Geometry check sheet. Reference: drawing and pictorial views, mm from the part's lowest x, y, z. A direction names the side the tool comes from. Coordinates: 2 decimals unless noted, no trailing zeros. Loops run counter-clockwise (first coordinate to the right, second up) from the corner with the lowest first, then second, coordinate; pieces in that order, holes last.
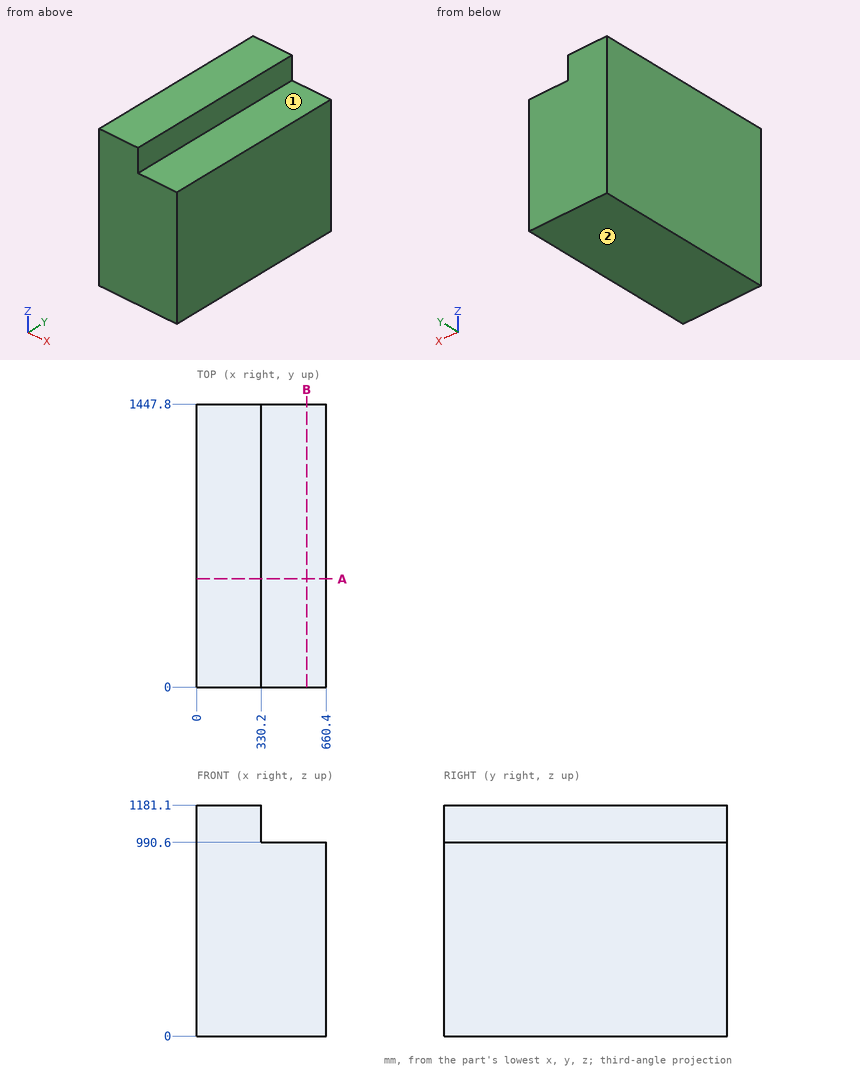
1) Access from +Z, -Z, +X, -X, +Y, -Y to the whole of each face (thin tool, end or side, straight path). Record for the marked faces 1 and 2.
Data:
face 1: +Z, +X, +Y, -Y
face 2: -Z, +X, -X, +Y, -Y
2) Section check A-A on y = 554. Record the cut outline in (x, z).
Data:
outline: (0, 0) - (660.4, 0) - (660.4, 990.6) - (330.2, 990.6) - (330.2, 1181.1) - (0, 1181.1) - close
3) Section check B-B on x = 561.5. Record the cut outline in (y, z).
Data:
outline: (0, 0) - (1447.8, 0) - (1447.8, 990.6) - (0, 990.6) - close
4) Material ranges on probe 1 along Z at (x, y) = (544.5, 662.5); probe 2 along X at (y, z) = (1313.5, 995), recorded low to high.
Data:
probe 1: z = 0 to 990.6
probe 2: x = 0 to 330.2
5) Depth check by flat-ended pin: pin 1 (12 mm diameter, centred on x = 247, y = 1087, fed in from -Z); pin 2 (3 mm diameter, centred on x = 462.5, y = 597, fed in from +Z). Enter the tip coordinate at first touch or a pass-through.
Data:
pin 1: stops at z = 0
pin 2: stops at z = 990.6
